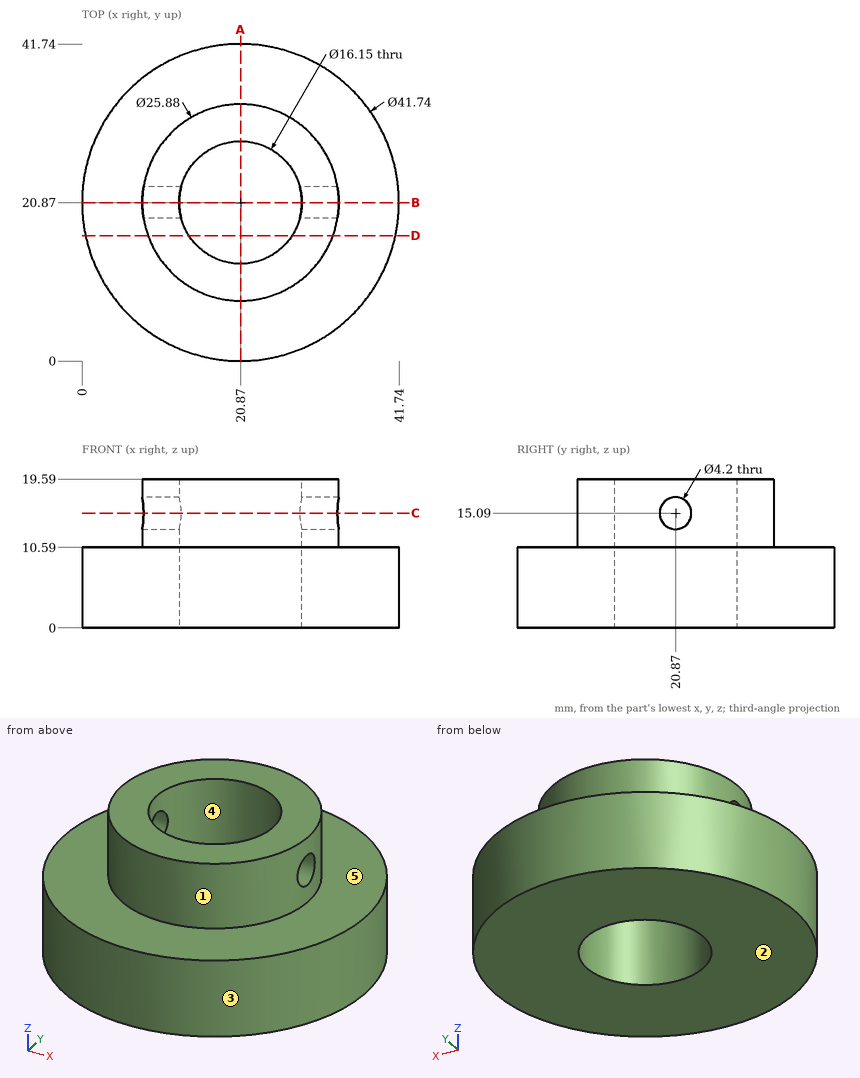
Verification items for this drawing (mm, ordinates from the low corner). A direction names the side the tool comes from. Coordinates: 2 decimals unless noted, no trailing zeros. Loops run counter-clockwise (first coordinate to the right, second up) from the corner with the lowest first, then second, coordinate; pieces in that order, holes last.
Item 1: Thickness scan on line 1 (Z direction, x = 32.75, y = 20.87); line 2 (Z direction, x = 21, y = 35); line 3 (X direction, y = 17, z = 9.5). Record the ranges inside material, lowest first.
Item 2: Release check for a two-part mould opening along X. For the marked faces 3, 4 and 5 record: released by +X, released by -X, zero draft, split by the parting line, or undercut.
Item 3: Access from +Z, -Z, +X, -X, +Y, -Y to the whole of each face (thin tool, end or side, straight path). Record for the marked faces 1 and 2.
Item 4: Sectioned sample at C-C, the plane z = 15.09. Record the boundary of the cut face in (x, y) (3 decimals), then the cut area to 3 significant figures.
Item 5: Sectioned sample at B-B, the plane y = 20.87. Record the boundary of the cut face in (x, z) (3 decimals), then the cut area to 3 significant figures.
Item 6: Go/stop test with flat-tipped pins: pin 1 Ø4 at (y, z) = (20.87, 15.09) entering from +X; pin 2 Ø3 at (x, y) = (5.5, 12.5) entering from +Z; pin 3 Ø1.5 at (y, z) = (25, 14) entering from +X; pin 4 Ø5 at (y, z) = (17.5, 10.5) entering from +X. Record where each tip stops, or that it passes through.
Item 7: Sectioned sample at A-A, the plane x = 20.87. Record the boundary of the cut face in (y, z) (3 decimals), then the cut area to 3 significant figures.
Item 8: Sectioned sample at D-D, the plane y = 16.5. Record the boundary of the cut face in (x, z).
Check result:
1. line 1: z = 0 to 12.99, 17.19 to 19.59
1. line 2: z = 0 to 10.59
1. line 3: x = 0.36 to 13.78, 27.96 to 41.38
2. face 3: split by the parting line
2. face 4: undercut
2. face 5: zero draft
3. face 1: +Z
3. face 2: -Z, +X, -X, +Y, -Y
4. outline: (8.102, 18.77) arc R12.94 ccw to (33.638, 18.77) - (28.667, 18.77) arc R8.075 cw to (13.073, 18.77) - close; (8.102, 22.97) - (13.073, 22.97) arc R8.075 cw to (28.667, 22.97) - (33.638, 22.97) arc R12.94 ccw to start
4. area: 280 mm2
5. outline: (0, 0) - (12.795, 0) - (12.795, 12.99) - (7.93, 12.99) - (7.93, 10.59) - (0, 10.59) - close; (7.93, 17.19) - (12.795, 17.19) - (12.795, 19.59) - (7.93, 19.59) - close; (28.945, 0) - (41.74, 0) - (41.74, 10.59) - (33.81, 10.59) - (33.81, 12.99) - (28.945, 12.99) - close; (28.945, 17.19) - (33.81, 17.19) - (33.81, 19.59) - (28.945, 19.59) - close
5. area: 318 mm2
6. pin 1: passes through
6. pin 2: stops at z = 10.59
6. pin 3: stops at x = 33.36
6. pin 4: stops at x = 41.72
7. outline: (0, 0) - (12.795, 0) - (12.795, 19.59) - (7.93, 19.59) - (7.93, 10.59) - (0, 10.59) - close; (28.945, 0) - (41.74, 0) - (41.74, 10.59) - (33.81, 10.59) - (33.81, 19.59) - (28.945, 19.59) - close
7. area: 359 mm2
8. outline: (0.46, 0) - (14.08, 0) - (14.08, 19.59) - (8.69, 19.59) - (8.69, 10.59) - (0.46, 10.59) - close; (27.66, 0) - (41.28, 0) - (41.28, 10.59) - (33.05, 10.59) - (33.05, 19.59) - (27.66, 19.59) - close
